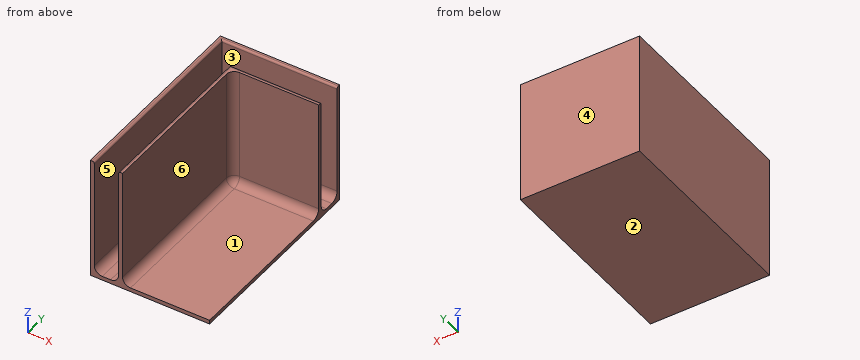
from build123d import *

# Parameters (mm, degrees)
SKETCH1_W           = 30
SKETCH1_H           = 50
BOSS_EXTRUDE1_DEPTH = 1
BOSS_EXTRUDE2_DEPTH = 30
FILLET1_R           = 2
FILLET2_R           = 0.5


with BuildPart() as part:
    # Sketch1 → Boss-Extrude1 (new body)
    with BuildSketch(Plane.XY):
        with Locations((15, 25)):
            Rectangle(SKETCH1_W, SKETCH1_H)
    extrude(amount=BOSS_EXTRUDE1_DEPTH)

    # Sketch2 → Boss-Extrude2 (add)
    with BuildSketch(Plane.XY.offset(1)):
        Polygon((0, 50), (30, 50), (30, 49), (1, 49), (1, 0), (0, 0), (0, 49), align=None)
        Polygon((30, 41.9), (8.1, 41.9), (8.1, 0), (7.1, 0), (7.1, 41.9), (7.1, 42.9), (30, 42.9), align=None)
    extrude(amount=BOSS_EXTRUDE2_DEPTH)

    # Fillet1
    fillet1_edges = [part.edges().sort_by_distance(p)[0] for p in [
        (1, 24.5, 1),
        (15.5, 49, 1),
        (18.55, 42.9, 1),
        (7.1, 21.45, 1),
        (8.1, 20.95, 1),
        (19.05, 41.9, 1),
        (8.1, 41.9, 16),
    ]]
    fillet(fillet1_edges, radius=FILLET1_R)

    # Fillet2
    fillet2_edges = [part.edges().sort_by_distance(p)[0] for p in [
        (1, 24.5, 31),
        (15.5, 49, 31),
        (18.55, 42.9, 31),
        (7.1, 21.45, 31),
    ]]
    fillet(fillet2_edges, radius=FILLET2_R)


solid = part.part
Geometry: final body of the model. Coordinates: model frame, mm. Face numbers are marked on the shaded views. A direction names the side the tool comes from. Coordinates: 2 decimals unless noted, no trailing zeros. Write each loop counter-clockwise with the first axis right and the second up, starting at its lowest first coordinate (ties: lowest second). Pieces come first, ordered by that corner, then holes. Notation, with made-up numbers: (38, -29.5) - (84, -29.5) arc R5 ccw to (84, -20.5) - close; hole circle Ø7 at (64.5, 58.25). An arc over 180 degrees is marked (long way). Return JSON: item names as keys, results as strings.
Item 1: Reachability of the marked faces 1, 2 and 3 from +Z, -Z, +X, -X, +Y, -Y: full face, straight path, thin tool, end or side. Return the list, or none.
Completed:
{"face 1": "+Z, +X, -Y", "face 2": "-Z, +X, -X, +Y, -Y", "face 3": "+Z, +X"}
Item 2: Line query: L1, parallel to X at y = 33.5, z = 16; L2, parallel to Y at x = 14.75, z = 13; L3, parallel to Z at x = 28.5, y = 27.5. Output: solid intervals per line, ascending.
Completed:
{"L1": "x = 0 to 1, 7.1 to 8.1", "L2": "y = 41.9 to 42.9, 49 to 50", "L3": "z = 0 to 1"}
Item 3: Section query B-B (y = 8.5). Output: boundary loops of the cut face in (x, z), and give its area (3 significant figures).
Completed:
{"outline": "(0, 0) - (30, 0) - (30, 1) - (10.1, 1) arc R2 cw to (8.1, 3) - (8.1, 31) - (7.6, 31) arc R0.5 ccw to (7.1, 30.5) - (7.1, 3) arc R2 cw to (5.1, 1) - (3, 1) arc R2 cw to (1, 3) - (1, 30.5) arc R0.5 ccw to (0.5, 31) - (0, 31) - close", "area": "92.5 mm2"}
Item 4: Pin query (flat end, axial travel): pin 1 Ø10 at (x, y) = (19.5, 20) entering from +Z; pin 2 Ø8 at (y, z) = (16, 27.5) entering from +X; pin 3 Ø1.5 at (x, z) = (23, 25.5) entering from -Y. Return the tip coordinate at first contact, or that it passes through.
Completed:
{"pin 1": "stops at z = 1", "pin 2": "stops at x = 8.1", "pin 3": "stops at y = 41.9"}
Item 5: Section query C-C (x = 27.75). Output: boundary loops of the cut face in (y, z).
Completed:
{"outline": "(0, 0) - (50, 0) - (50, 31) - (49.5, 31) arc R0.5 ccw to (49, 30.5) - (49, 3) arc R2 cw to (47, 1) - (44.9, 1) arc R2 cw to (42.9, 3) - (42.9, 30.5) arc R0.5 ccw to (42.4, 31) - (41.9, 31) - (41.9, 3) arc R2 cw to (39.9, 1) - (0, 1) - close"}
Item 6: Section query A-A (z = 21). Output: boundary loops of the cut face in (x, y), and give its area (3 significant figures).
Completed:
{"outline": "(0, 0) - (1, 0) - (1, 49) - (30, 49) - (30, 50) - (0, 50) - close; (7.1, 0) - (8.1, 0) - (8.1, 39.9) arc R2 cw to (10.1, 41.9) - (30, 41.9) - (30, 42.9) - (7.1, 42.9) - close", "area": "145 mm2"}
Item 7: Pull-direction query (X, two-part tool) for the marked faces 4, 5 and 6; classes: +X half, -X half, draft (parallel to the pull), parting line (faces both ways), or undercut.
Completed:
{"face 4": "draft", "face 5": "undercut", "face 6": "+X half"}
